Design review of the part built by this model. Coordinates are the model's own, in mm. Give positions to 0.01 mm unless a question says otherwise; leave off trailing zeros. Order: outer loops, then holes, each group sorted by start corner. A loop starts at its lowest first (then second) coordinate and runs counter-clockwise, first axis right, second up. Notation, with made-up numbers: M -21,80 L 14,80 A19 ccw 14,110 Z; hole C 58.25,-39.5 d11. An arc over 180 degrees is marked long. Answer as a JSON object with one key per item and string values.
from build123d import *

# Parameters (mm, degrees)
BOSS_EXTRU_1_DEPTH = 3
CONG_1_R           = 10


with BuildPart() as part:
    # Esquisse1 → Boss.-Extru.1 (new body)
    with BuildSketch(Plane.XY):
        Polygon((11.917194627, -65.85290432), (11.917194627, -10.85290432), (2.917194627, -10.85290432), (2.917194627, -65.85290432), (-10.53158391, -34.67577833), (-31.222461176, -23.509273139), (-34.178300785, 10.64709568), (49.012690039, 10.64709568), (46.05685043, -23.509273139), (25.365973164, -34.67577833), align=None)
    extrude(amount=BOSS_EXTRU_1_DEPTH)

    # Congé1
    cong_1_edges = [part.edges().sort_by_distance(p)[0] for p in [
        (-10.53158391, -34.67577833, 1.5),
        (-31.222461176, -23.509273139, 1.5),
        (46.05685043, -23.509273139, 1.5),
        (25.365973164, -34.67577833, 1.5),
    ]]
    fillet(cong_1_edges, radius=CONG_1_R)


solid = part.part
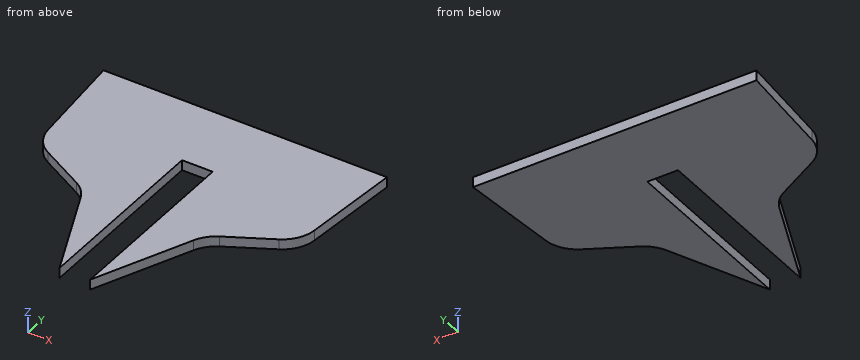
(1) We need section D-D (x = -23.5). Write out the cut boundary in (y, z), plus the area to 3 significant figures.
Checked values:
{"outline": "M -27.68,0 L 10.65,0 L 10.65,3 L -27.68,3 Z", "area": "115 mm^2"}
(2) We need section C-C (y = -42.5). Write out the cut boundary in (x, z), plus the area to 3 significant figures.
Checked values:
{"outline": "M -7.16,0 L 2.92,0 L 2.92,3 L -7.16,3 Z; M 11.92,0 L 21.99,0 L 21.99,3 L 11.92,3 Z", "area": "60.4 mm^2"}
(3) We need section A-A (y = -13). Write out the cut boundary in (x, z).
Checked values:
{"outline": "M -32.13,0 L 2.92,0 L 2.92,3 L -32.13,3 Z; M 11.92,0 L 46.97,0 L 46.97,3 L 11.92,3 Z"}
(4) To check wall thickness, follow L1, parallel to Y at x = 5, z = 0.9; L2, parallel to X at y = -55.5, z = 1.4; L3, parallel to X at y = -27.5, z = 0.7. State the ranges of each line that lie inside material, in increasing order. Write a range as from..to.
Checked values:
{"L1": "y = -10.85..10.65", "L2": "x = -1.55..2.92, 11.92..16.38", "L3": "x = -23.83..2.92, 11.92..38.66"}
(5) We need section B-B (z = 1.45). Write out the cut boundary in (x, y), plus the area to 3 significant figures.
Checked values:
{"outline": "M -34.18,10.65 L -31.69,-18.13 A10 ccw -26.47,-26.07 L -13.59,-33.03 A10 cw -9.16,-37.87 L 2.92,-65.85 L 2.92,-10.85 L 11.92,-10.85 L 11.92,-65.85 L 23.99,-37.87 A10 cw 28.42,-33.03 L 41.31,-26.07 A10 ccw 46.52,-18.13 L 49.01,10.65 Z", "area": "3,570 mm^2"}
(6) Insertion check: pin 1 (0.9 mm diameter, centred on y = -40.5, z = 1.5, fed in from -X); pin 2 (1.5 mm diameter, centred on x = 4.5, z = 2, fed in from -Y); pin 3 (1 mm diameter, centred on y = -3, z = 2.5, fed in from +X); pin 4 (10 mm diameter, centred on x = 5, y = -31.5, fed in from -Z). Each pin has a flat end and moves straight along its axis. Give the tip position at first contact, or say it passes through.
Checked values:
{"pin 1": "stops at x = -8.21", "pin 2": "stops at y = -10.85", "pin 3": "stops at x = 47.87", "pin 4": "stops at z = 0"}
